The model under review builds one solid part; all positions refer to its coordinate system, in mm. A direction names the side the tool comes from. Give positions to 0.01 mm unless a question says otherwise; leave off trailing zeros. Loops run counter-clockwise (first coordinate to the right, second up) from the corner with the lowest first, then second, coordinate; pieces in that order, holes last. Notation, with made-up numbers: M -17.75,81 L -8.75,81 A20 ccw -8.75,106 Z; hole C 81.25,-13 d7. An arc over 180 degrees is marked long. Put each result on its own line as item: value. Start each with the question number.
from build123d import *

# Parameters (mm, degrees)
CYLINDER023_R     = 2.5
CYLINDER023_DEPTH = 7.5
CYLINDER022_R     = 2.5
CYLINDER022_DEPTH = 7.5
EXTRUDE001_DEPTH  = 4


with BuildPart() as cilindro018:
    # Cylinder023 → Cylinder023 (new body)
    with BuildSketch(Plane(origin=(27.5, 12, 5), x_dir=(1, 0, 0), z_dir=(0, 0, 1))):
        Circle(CYLINDER023_R)
    extrude(amount=CYLINDER023_DEPTH)


with BuildPart() as fusion011:
    # Cylinder022 → Cylinder022 (new body)
    with BuildSketch(Plane(origin=(-27.5, 12, 5), x_dir=(1, 0, 0), z_dir=(0, 0, 1))):
        Circle(CYLINDER022_R)
    extrude(amount=CYLINDER022_DEPTH)

    # Fusion011: union Cilindro018
    add(cilindro018.part)


with BuildPart() as cut005:
    # Sketch006 (on Face2 of Cylinder008) → Extrude001 (new body)
    with BuildSketch(Plane(origin=(0, 12, 1.5), x_dir=(1, 0, 0), z_dir=(0, 0, 1))):
        with BuildLine():
            ThreePointArc((23.5, 0), (27.5, -4), (31.5, 0))
            Line((31.5, 0), (31.5, 4.555666))
            ThreePointArc((31.5, 4.555666), (0, 24.29952), (-31.5, 4.555666))
            Line((-31.5, 0), (-31.5, 4.555666))
            ThreePointArc((-31.5, 0), (-27.5, -4), (-23.5, 0))
            Line((-23.5, 0), (-23.5, 2.594256))
            ThreePointArc((23.5, 2.594256), (0, 16.29952), (-23.5, 2.594256))
            Line((23.5, 0), (23.5, 2.594256))
        make_face()
    extrude(amount=EXTRUDE001_DEPTH)


with BuildPart() as cut005_1:
    # Extrude001 placement: moved
    add(cut005.part.moved(Location((0, 0, 5))))

    # Cut005: cut Fusion011
    add(fusion011.part, mode=Mode.SUBTRACT)


solid = cut005_1.part
(1) We need section D-D, the plane y = 25. Write out the cut boundary in (x, z).
(2) We need section A-A, the plane z = 9.9. Write out the cut boundary in (x, y).
(3) For faces 4 (the cylindrical face through (-28.04, 9.56, 8.47)), 5 (the flat face through (-23.5, 13, 8)), list the 3-axis set-ups (+Z, -Z, +X, -X, +Y, -Y) from which the entire face can be reached by the end or side of a thin tool; tool diameter is ignored.
(4) To check wall thickness, follow L1, parallel to X at y = 12, z = 7.7; L2, parallel to X at y = 25, z = 9.4; L3, parallel to X at y = 15, z = 6.7. State the ranges of each line that lie inside material, in increasing order. Write a range as [from, to].
(5) Insertion check: pin 1 (1 mm diameter, centred on x = -14, z = 10, fed in from -Y); pin 2 (3 mm diameter, centred on x = -27.5, y = 12, fed in from +Z); pin 3 (1.5 mm diameter, centred on y = 23, z = 8.5, fed in from -X). Each pin has a flat end and moves straight along its axis. Give the tip position at first contact, or say it passes through.
(6) We need section C-C, the plane x = -27.5. Write out the cut boundary in (y, z), plus the area to 3 significant figures.
(7) We need section B-B, the plane y = 13. Write out the cut boundary in (x, z).
(8) Draft analysis for pull direction X (two halves, no side actions). For faces 1 (the flat face through (31.5, 14, 8)), 2 (the flat face through (2, 29, 10.5)), 3 (the cylindrical face through (-27.6, 8, 8.5)), state which applies: +X half, -X half, draft (parallel to the pull), parting line (faces both ways), or undercut.
Check sheet entries:
1. outline: M -25.75,6.5 L -12.93,6.5 L -12.93,10.5 L -25.75,10.5 Z; M 12.93,6.5 L 25.75,6.5 L 25.75,10.5 L 12.93,10.5 Z
2. outline: M -31.5,12 A4 ccw -23.5,12 L -23.5,14.59 A27 cw 23.5,14.59 L 23.5,12 A4 ccw 31.5,12 L 31.5,16.56 A35 ccw -31.5,16.56 Z; hole C -27.5,12 d5; hole C 27.5,12 d5
3. face 4: +Z, -Z
3. face 5: +Z, -Z, -Y
4. L1: x = [-31.5, -30], [-25, -23.5], [23.5, 25], [30, 31.5]
4. L2: x = [-25.75, -12.93], [12.93, 25.75]
4. L3: x = [-31.5, -23.27], [23.27, 31.5]
5. pin 1: stops at y = 24.08
5. pin 2: passes through
5. pin 3: stops at x = -28.04
6. outline: M 8,6.5 L 9.5,6.5 L 9.5,10.5 L 8,10.5 Z; M 14.5,6.5 L 22.95,6.5 L 22.95,10.5 L 14.5,10.5 Z
6. area: 39.8 mm²
7. outline: M -31.5,6.5 L -29.79,6.5 L -29.79,10.5 L -31.5,10.5 Z; M -25.21,6.5 L -23.5,6.5 L -23.5,10.5 L -25.21,10.5 Z; M 23.5,6.5 L 25.21,6.5 L 25.21,10.5 L 23.5,10.5 Z; M 29.79,6.5 L 31.5,6.5 L 31.5,10.5 L 29.79,10.5 Z
8. face 1: +X half
8. face 2: draft
8. face 3: undercut
